Input: part model. Units: mm. Frame: model coordinates. Face numbers are marked on the shaded views. A direction names the side the tool comes from. Give positions to 0.01 mm unless a question says otherwise; leave off trailing zeros. Order: outer loops, then holes, each group sorted by start corner. A loop starts at its lowest first (then second) coordinate and runs counter-clockwise, first axis right, second up. Notation, with made-up numbers: (51.25, -17) - (57.25, -17) arc R31 cw to (57.25, 22) - close; hole circle Ø1 at (35, 70.25). An arc over 180 degrees is marked (long way). Answer in a Markdown table with one row per item. Add a question column.
1. Section query B-B on y = -42. Return loops of the section in (x, z), and give its area (3 significant figures).
2. Section query A-A on y = -10. Return loops of the section in (x, z), and give its area (3 significant figures).
3. Contact query for flat-ended pins moving along their axis: pin 1 (5 mm diameter, centred on x = 42, y = 7, fed in from -Z); pin 2 (0.9 mm diameter, centred on y = -19.5, z = -2, fed in from +X); pin 3 (2.5 mm diameter, centred on x = 5, y = -62, fed in from +Z). Output: stop coordinate, or through.
4. Ray query, line 1 (X direction, y = -10, z = 0.05); line 2 (X direction, y = -10, z = -0.8); line 3 (Z direction, x = 39.5, y = -57). Return the intervals inside material, ascending. Write a range as [from, to].
5. Access query for the marked faces 1 and 2. Directions: +Z, -Z, +X, -X, +Y, -Y. A direction counts if a zero-diameter tool reaches every point of the face in a straight line with its end or side. Return the directions, or none.
6. Section query C-C on x = 60.5. Return loops of the section in (y, z), and give its area (3 significant figures).
7. Section query D-D on z = -1.05. Return loops of the section in (x, y), and give its area (3 significant figures).
Autodesk Inventor part; units mm, degrees
ref_plane "Plano de trabajo7" through (63.9999, 14.8405, -83) normal (1, 0, 0) x (0, 1, 0)
ref_plane "Plano de trabajo6" through (9.9999, -67, -72) normal (0, 0, 1) x (1, 0, 0)
ref_plane "YZ Plane" through (0, 0, 0) normal (1, 0, 0) x (0, 1, 0)
ref_plane "Plano de trabajo7" through (63.9999, 14.8405, -83) normal (1, 0, 0) x (0, 1, 0)
sketch "Boceto2" plane through (0, 0, 0) normal (1, 0, 0) x (0, 1, 0)
  line L0 (0, 0) -> (-67, 0)
  line L1 (-67, 0) -> (-67, 3)
  line L2 (-67, 3) -> (0, 3)
  line L3 (0, 3) -> (0, 0)
  line L4 (16.65, -80) -> (16.65, 9)
  line L5 (0, 3) -> (16.65, 3)
  line L6 (16.65, 3) -> (16.65, 0)
  line L7 (16.65, 0) -> (0, 0)
  line L8 (0, 0) -> (0, 3)
  dimension "d2" = 67
  dimension "d3" = 3
extrude "Extrusión2" add sketch "Boceto2" along normal up to surface (63.9999 mm away)
sketch "Boceto8" plane through (0, -67, 3) normal (0, 0, 1) x (1, 0, 0)
  circle A0 centre (4.9999, 5) radius 2.1
  circle A1 centre (4.9999, 57) radius 2.1
  line L0 (-2.0001, 83.65) -> (-2.0001, 76.5)
  line L1 (-2.0001, 76.5) -> (-20.0001, 76.5)
  line L2 (-20.0001, 76.5) -> (-20.0001, 0)
  line L3 (9.9999, 0) -> (-20.0001, 0)
  line L4 (9.9999, 0) -> (9.9999, 83.65)
  line L5 (9.9999, 83.65) -> (-2.0001, 83.65)
  circle A2 centre (4.9999, 57) radius 1.6
  circle A3 centre (4.9999, 5) radius 1.6
  point P0 (0, 67)
  dimension "d31" = 3.2
  dimension "d32" = 3.2
hole "Agujero3" at (4.9999, -10, 3) at (4.9999, -62, 3) direction (0, 0, -1) diameter 3.2 depth 5
sketch "Boceto9" plane through (0, -67, 0) normal (0, 0, -1) x (-1, 0, 0)
  line L0 (-9.9999, 83.65) -> (-9.9999, 0)
  line L1 (-63.9999, 0) -> (-9.9999, 0)
  circle A0 centre (-4.9999, 5) radius 1.6
  circle A1 centre (-4.9999, 57) radius 1.6
  line L2 (0, 0) -> (0, 83.65)
  line L3 (0, 83.65) -> (-63.9999, 83.65)
  line L4 (0, 0) -> (-63.9999, 0)
  line L5 (-63.9999, 83.65) -> (-63.9999, 0)
  line L6 (-9.9999, 83.65) -> (-32.9722, 83.65)
  line L7 (-40.0761, 83.65) -> (-63.9999, 83.65)
  line L8 (-32.9722, 83.65) -> (-29.7863, 64.5577)
  line L9 (-34.4654, 63.5184) -> (-40.0761, 83.65)
  arc A2 (-34.4654, 63.5184) -> (-29.7863, 64.5577) centre (-32.1535, 64.1627) ccw
  line L10 (-63.9999, 83.65) -> (-63.9999, 0)
  point P0 (0, 67)
  point P1 (-63.9999, 0)
  point P2 (-37.9999, 83.65)
extrude "Extrusión6" add sketch "Boceto9" along normal blind 3 contours L3 L2 L4 L0
sketch "Boceto10" plane through (65, -67, 0) normal (0, 0, -1) x (-1, 0, 0)
  line L0 (24.0001, 83.65) -> (24.0001, 86.65)
  line L1 (24.0001, 83.65) -> (27.0001, 83.65)
  line L2 (65, 83.65) -> (1.0001, 83.65)
  line L3 (35.8799, 60.5564) -> (35.8799, 64.1631)
  line L4 (35.8799, 60.4) -> (35.8799, 60.5564)
  line L5 (35.8799, 60.4) -> (33.8799, 60.4)
  line L6 (27.0001, 83.65) -> (30.0001, 83.65)
  line L7 (30.0001, 83.65) -> (33.8799, 60.4)
  line L8 (33.8799, 60.4) -> (33.4799, 60.4)
  line L9 (33.4799, 60.4) -> (27.0001, 83.65)
  point P0 (65, 67)
  point P1 (0, 83.65)
  dimension "d42" = 3
  dimension "d43" = 2
  dimension "d44" = 3
  dimension "d48" = 0.4
ref_plane "Plano de trabajo6" through (9.9999, -67, -72) normal (0, 0, 1) x (1, 0, 0)
extrude "Extrusión7" [suppressed]
fillet "Empalme1" [suppressed]
fillet "Empalme2" [suppressed]
properties part number "Lateral derecho"
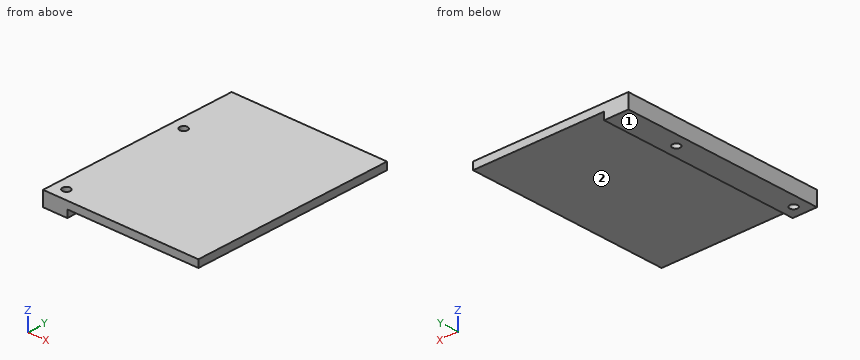
Answer:
| question | item | result |
|---|---|---|
| 1 | outline | (0, -3) - (10, -3) - (10, 0) - (64, 0) - (64, 3) - (0, 3) - close |
| 1 | area | 222 mm² |
| 2 | outline | (0, -3) - (3.4, -3) - (3.4, 3) - (0, 3) - close; (6.6, -3) - (10, -3) - (10, 0) - (64, 0) - (64, 3) - (6.6, 3) - close |
| 2 | area | 203 mm² |
| 3 | pin 1 | stops at z = 0 |
| 3 | pin 2 | stops at x = 10 |
| 3 | pin 3 | passes through |
| 4 | line 1 | x = [0, 3.4], [6.6, 64] |
| 4 | line 2 | x = [0, 3.4], [6.6, 10] |
| 4 | line 3 | z = [0, 3] |
| 5 | face 1 | -Z, +X, -X, +Y, -Y |
| 5 | face 2 | -Z, +X, +Y, -Y |
| 6 | outline | (-67, 0) - (16.65, 0) - (16.65, 3) - (-67, 3) - close |
| 6 | area | 251 mm² |
| 7 | outline | (0, -67) - (10, -67) - (10, 16.65) - (0, 16.65) - close; hole circle Ø3.2 at (5, -62); hole circle Ø3.2 at (5, -10) |
| 7 | area | 820 mm² |
